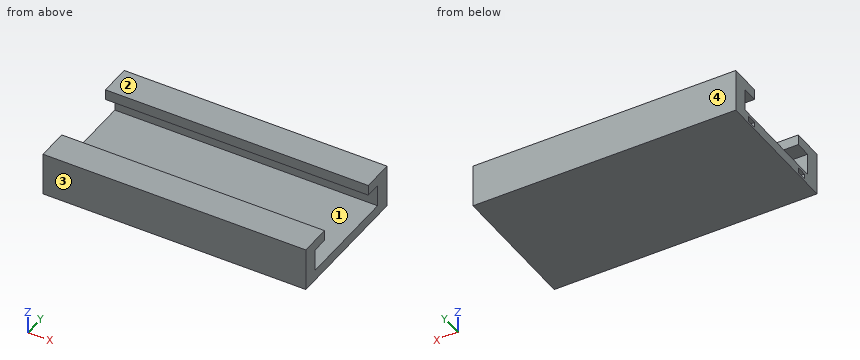
Autodesk Inventor part; units mm, degrees
ref_plane "YZ Plane" through (0, 0, 0) normal (1, 0, 0) x (0, 1, 0)
ref_plane "XZ Plane" through (0, 0, 0) normal (0, 1, 0) x (-1, 0, 0)
ref_plane "XY Plane" through (0, 0, 0) normal (0, 0, 1) x (1, 0, 0)
sketch "Sketch1" plane through (0, 0, 0) normal (0, 0, 1) x (1, 0, 0)
  line L0 (-114.7642, 55) -> (135.2358, 55)
  line L1 (135.2358, 55) -> (135.2358, -75)
  line L2 (135.2358, -75) -> (-114.7642, -75)
  line L3 (-114.7642, -75) -> (-114.7642, 55)
  point P0 (0, 0)
  dimension "d0" = 250
  dimension "d1" = 130
extrude "Extrusion1" add sketch "Sketch1" along normal blind 10
sketch "Sketch2" plane through (0, 0, 10) normal (0, 0, 1) x (1, 0, 0)
  line L0 (135.2358, 55) -> (-114.7642, 55)
  line L1 (135.2358, -75) -> (135.2358, 55)
  line L2 (-114.7642, 55) -> (135.2358, 55)
  line L3 (135.2358, 55) -> (135.2358, 40)
  line L4 (135.2358, 40) -> (-114.7642, 40)
  line L5 (-114.7642, 40) -> (-114.7642, 55)
  line L6 (-114.7642, -75) -> (135.2358, -75)
  line L7 (135.2358, -75) -> (135.2358, -60)
  line L8 (135.2358, -60) -> (-114.7642, -60)
  line L9 (-114.7642, -60) -> (-114.7642, -75)
  point P0 (0, 0)
  dimension "d4" = 15
  dimension "d5" = 15
extrude "Extrusion2" add sketch "Sketch2" along normal blind 21
sketch "Sketch3" plane through (0, 0, 31) normal (0, 0, 1) x (1, 0, 0)
  line L0 (-114.7642, 55) -> (-114.7642, -75)
  line L1 (135.2358, -60) -> (135.2358, 40)
  line L2 (-114.7642, 55) -> (135.2358, 55)
  line L3 (135.2358, 55) -> (135.2358, 25)
  line L4 (135.2358, 25) -> (-114.7642, 25)
  line L5 (-114.7642, 25) -> (-114.7642, 55)
  line L6 (135.2358, -75) -> (135.2358, -60)
  line L7 (135.2358, -75) -> (-114.7642, -75)
  line L8 (-114.7642, -75) -> (-114.7642, -45)
  line L9 (-114.7642, -45) -> (135.2358, -45)
  line L10 (135.2358, -45) -> (135.2358, -75)
  point P0 (0, 0)
  point P1 (-114.7642, -45)
  dimension "d8" = 30
  dimension "d9" = 30
extrude "Extrusion3" add sketch "Sketch3" along normal blind 10 contours L2 L3 L1 L4 L0 | L9 L1 L6 L7 L0
sketch "Sketch4" plane through (-114.7642, -75, 0) normal (-1, 0, 0) x (0, 0, 1)
  line L0 (7.1242, 110) -> (2.1242, 110)
  line L1 (2.1242, 110) -> (2.1242, 100)
  line L2 (2.1242, 100) -> (7.1242, 100)
  line L3 (7.1242, 100) -> (7.1242, 110)
  line L4 (7.1242, 30) -> (2.1242, 30)
  line L5 (2.1242, 30) -> (2.1242, 20)
  line L6 (2.1242, 20) -> (7.1242, 20)
  line L7 (7.1242, 20) -> (7.1242, 30)
  line L8 (31, 100) -> (41, 100)
  line L9 (31, 30) -> (41, 30)
  point P0 (0, 75)
  dimension "d12" = 5
  dimension "d13" = 10
  dimension "d14" = 10
  dimension "d15" = 0
  dimension "d16" = 0
extrude "Extrusion4" cut sketch "Sketch4" against normal blind 20
equation "\"d5\" = d4"
equation "\"d9\" = d8"
properties part number "Part1_with_things"
Here's how the part is built. I have some questions about the finished solid (model axes, mm). Face numbers are marked on the shaded views. Give positions to 0.01 mm unless a question says otherwise; leave off trailing zeros. Loops run counter-clockwise (first coordinate to the right, second up) from the corner with the lowest first, then second, coordinate; pieces in that order, holes last. Notation, with made-up numbers: (-19, 56) -> (35, 56) arc R8 cw to (35, 68) -> close; hole circle Ø5 at (34.5, 47). An arc over 180 degrees is marked (long way). Answer as a JSON object with one key per item and string values. Group by question number.
Item 1: Imagine slicing it at A-A on z = 34.5. Write out the boundary of the cut face in (x, y), then the cut area to 3 significant figures.
Item 2: Imagine slicing it at B-B on y = 30. Write out the boundary of the cut face in (x, z), then the cut area to 3 significant figures.
Item 3: Thinking about a two-plate mould opening in Y: for the marked faces 1, 2, 3 and 4, which applies, pulls with the +Y half, pulls with the -Y half, needs draft (parallel to the pull), parting line crosses it, or undercut?
Item 4: I need wall thicknesses on L1, parallel to Y at x = 10, z = 28.5; L2, parallel to Z at x = 75, y = 16; L3, parallel to X at y = -51.5, z = 7. Which ranges of each line are inside material? Lowest first, please.
Item 5: Will these pins go through, and if not, where does the flat tip stop? pin 1 (3 mm diameter, centred on x = -105, y = 30, fed in from -Z); pin 2 (2 mm diameter, centred on x = -84.5, y = -10, fed in from +Z); pin 3 (1.5 mm diameter, centred on y = 27.5, z = 4.5, fed in from -X); pin 4 (10 mm diameter, centred on y = -17.5, z = 18, fed in from -X) (1 decimal).
Item 6: Imagine slicing it at C-C on x = -64. Write out the boundary of the cut face in (y, z), then the cut area to 3 significant figures.
Answer list:
{
 "1": {"outline": "(-114.76, -75) -> (135.24, -75) -> (135.24, -45) -> (-114.76, -45) -> close; (-114.76, 25) -> (135.24, 25) -> (135.24, 55) -> (-114.76, 55) -> close", "area": "15,000 mm2"},
 "2": {"outline": "(-114.76, 0) -> (135.24, 0) -> (135.24, 10) -> (-114.76, 10) -> (-114.76, 7.12) -> (-94.76, 7.12) -> (-94.76, 2.12) -> (-114.76, 2.12) -> close; (-114.76, 31) -> (135.24, 31) -> (135.24, 41) -> (-114.76, 41) -> close", "area": "4,900 mm2"},
 "3": {"face 1": "undercut", "face 2": "needs draft", "face 3": "pulls with the -Y half", "face 4": "pulls with the +Y half"},
 "4": {"L1": "y = -75 to -60, 40 to 55", "L2": "z = 0 to 10", "L3": "x = -94.76 to 135.24"},
 "5": {"pin 1": "stops at z = 0", "pin 2": "stops at z = 10", "pin 3": "stops at x = -94.76", "pin 4": "passes through"},
 "6": {"outline": "(-75, 0) -> (55, 0) -> (55, 41) -> (25, 41) -> (25, 31) -> (40, 31) -> (40, 10) -> (-60, 10) -> (-60, 31) -> (-45, 31) -> (-45, 41) -> (-75, 41) -> close", "area": "2,530 mm2"}
}
